Design review of the part built by this model. Coordinates are the model's own, in mm. A direction names the side the tool comes from. Give positions to 0.01 mm unless a question says otherwise; leave off trailing zeros. Loops run counter-clockwise (first coordinate to the right, second up) from the corner with the lowest first, then second, coordinate; pieces in that order, holes last. Notation, with made-up numbers: (47, -2.5) -> (89, -2.5) arc R20 ccw to (89, 30.5) -> close; hole circle Ø5 at (46.25, 40). An arc over 180 degrees is marked (long way). Answer as CSV lines item,"result".
from build123d import *

# Parameters (mm, degrees)
F1_DEPTH = 60
F2_SIZE  = 3


with BuildPart() as f1:
    # F0 (on Top) → F1 (new body)
    with BuildSketch(Plane.XY):
        Polygon((57.207322, 5.764956), (-52.792678, 5.764956), (-52.792678, -18.955044), (-23.39, -18.955044), (-6.900156, -24.632953), (3.948288, -19.341813), (18.594371, -24.384864), (57.207322, -24.235044), align=None)
    extrude(amount=F1_DEPTH)

    # F2
    f2_edges = [f1.edges().sort_by_distance(p)[0] for p in [
        (-52.792678, -6.595044, 60),
        (-52.792678, -6.595044, 0),
        (57.207322, -9.235044, 60),
        (57.207322, -9.235044, 0),
    ]]
    chamfer(f2_edges, length=F2_SIZE)


solid = f1.part
Q1. We need section C-C, the plane x = 9.5. State the section outline as (y, z) points, and give its area (3 significant figures).
Filled sheet:
outline,"(-21.25, 0) -> (5.76, 0) -> (5.76, 60) -> (-21.25, 60) -> close"
area,"1,620 mm^2"
Q2. Clearance check with flat-ended pins moving along their axes: pin 1 Ø23.5 at (x, z) = (-37.5, 35) entering from -Y; pin 2 Ø3 at (x, z) = (1.5, 10.5) entering from -Y. State where each tip first meets the part, or that it passes through.
Filled sheet:
pin 1,"stops at y = -18.96"
pin 2,"stops at y = -21.27"
Q3. We need section B-B, the plane x = -38. State the section outline as (y, z) points, and give its area (3 significant figures).
Filled sheet:
outline,"(-18.96, 0) -> (5.76, 0) -> (5.76, 60) -> (-18.96, 60) -> close"
area,"1,480 mm^2"
Q4. We need section A-A, the plane z = 22. State the section outline as (x, y) points.
Filled sheet:
outline,"(-52.79, -18.96) -> (-23.39, -18.96) -> (-6.9, -24.63) -> (3.95, -19.34) -> (18.59, -24.38) -> (57.21, -24.24) -> (57.21, 5.76) -> (-52.79, 5.76) -> close"
Q5. For faces 1 (the flat face through (-1.552, -22.024, 29.58)), 2 (the flat face through (1, -9, 60)), 3 (the flat face through (-38, -18.955, 30)), list the 3-axis set-ups (+Z, -Z, +X, -X, +Y, -Y) from which the entire face can be reached by the end or side of a thin tool; tool diameter is ignored.
Filled sheet:
face 1,"+Z, -Z, -Y"
face 2,"+Z, +X, -X, +Y, -Y"
face 3,"+Z, -Z, -X, -Y"
Q6. To check wall thickness, follow probe 1 along Y at (x, z) = (-39.5, 40); probe 2 along Y at (x, z) = (21, 32.5). State the ranges of each line that lie inside material, in increasing order. Write a range as from..to.
Filled sheet:
probe 1,"y = -18.96..5.76"
probe 2,"y = -24.38..5.76"
Q7. The part is to be moulded in two halves that separate along X. For faces 4 (the flat face through (57.207, -9, 30)), 5 (the flat face through (3, 5.765, 30)), 6 (the flat face through (11.17, -21.83, 29.58)), 7 (the flat face through (-15.261, -21.754, 29.58)), say which applies: pulls with the +X half, pulls with the -X half, needs draft (parallel to the pull), parting line crosses it, or undercut.
Filled sheet:
face 4,"pulls with the +X half"
face 5,"needs draft"
face 6,"undercut"
face 7,"pulls with the -X half"
